Source: CAD feature listing. Evaluate the final solid. Frame: model axes, mm. A direction names the side the tool comes from. Give positions to 0.01 mm unless a question says otherwise; leave off trailing zeros. Write each loop counter-clockwise with the first axis right and the second up, starting at its lowest first coordinate (ties: lowest second). Pieces come first, ordered by that corner, then holes. Notation, with made-up numbers: M -6,-25 L 42,-25 A19 cw 42,3 Z; hole C 74.25,69.25 d10. An arc over 180 degrees is marked long. Return JSON: item names as keys, results as strings.
```python
from build123d import *

# Parameters (mm, degrees)
F1_DEPTH = 3.81
F3_DEPTH = 25.4
F4_R     = 8.724849
F5_DEPTH = 6.35
F7_D     = 15.24


with BuildPart() as f1:
    # F0 (on Top) → F1 (new body)
    with BuildSketch(Plane.XY):
        Polygon((-39.496768, 41.965317), (-39.496768, 35.576135), (-39.496768, -57.938274), (45.595534, -57.938274), (45.595534, 5.372723), (31.655498, 5.372723), (31.655498, 22.507351), (45.595534, 22.507351), (45.595534, 41.965317), align=None)
    extrude(amount=F1_DEPTH)

    # F2 (on face) → F3 (join)
    with BuildSketch(Plane.XY.offset(3.81)):
        Polygon((45.595534, 41.965317), (-39.496768, 41.965317), (-39.496768, -57.938274), (-29.332161, -57.938274), (-29.332161, -15.246916), (45.595534, -15.246916), (45.595534, 5.372723), (31.655498, 5.372723), (31.655498, 22.507351), (45.595534, 22.507351), align=None)
    extrude(amount=F3_DEPTH)

    # F4 (on face) → F5 (join)
    with BuildSketch(Plane.YZ.offset(-29.332161)):
        with Locations((-41.252476, 16.706923)):
            Circle(F4_R)
    extrude(amount=F5_DEPTH)

    # F7 (through all)
    with Locations(Plane.XZ.offset(15.246916)):
        with Locations((21.842908, 16.264843)):
            Hole(F7_D / 2)


solid = f1.part
```
1) Contact query for flat-ended pins moving along their axis: pin 1 Ø6 at (x, z) = (5, 21) entering from -Y; pin 2 Ø8 at (x, y) = (29.5, -37) entering from +Z; pin 3 Ø14 at (y, z) = (-42.5, 17.5) entering from +X. Output: stop coordinate, or through.
Numbers:
{"pin 1": "stops at y = -15.25", "pin 2": "stops at z = 3.81", "pin 3": "stops at x = -22.98"}
2) Cut plane A-A, the plane z = 5.75. Return the cut outline in (x, y).
Numbers:
{"outline": "M -39.5,-57.94 L -29.33,-57.94 L -29.33,-15.25 L 45.6,-15.25 L 45.6,5.37 L 31.66,5.37 L 31.66,22.51 L 45.6,22.51 L 45.6,41.97 L -39.5,41.97 Z"}
3) Set-up query: faces 1 (the face through (-13, -57.938, 3)), 2 (the face through (-22.982, -41, 17)), 3 (the face through (39, 5.373, 14)). Return all of +Z, -Z, +X, -X, +Y, -Y with unobstructed straight access to the full face (end or side cutting, diameter ignored); none if empty.
Numbers:
{"face 1": "+Z, -Z, +X, -X, -Y", "face 2": "+Z, +X, -Y", "face 3": "+Z, -Z, +X"}
4) Cut plane D-D, the plane z = 11. Return the cut outline in (x, y), then the cut area to 3 significant figures.
Numbers:
{"outline": "M -39.5,-57.94 L -29.33,-57.94 L -29.33,-47.85 L -22.98,-47.85 L -22.98,-34.65 L -29.33,-34.65 L -29.33,-15.25 L 16.33,-15.25 L 16.33,41.97 L -39.5,41.97 Z; M 27.35,-15.25 L 45.6,-15.25 L 45.6,5.37 L 31.66,5.37 L 31.66,22.51 L 45.6,22.51 L 45.6,41.97 L 27.35,41.97 Z", "area": "4,520 mm²"}
5) Line query: line 1 (Y direction, x = 37, z = 18.75); line 2 (X direction, y = -39.5, z = 13.75); line 3 (Y direction, x = 11.5, z = 22.25). Output: solid intervals per line, ascending. Write a range as [from, to].
Numbers:
{"line 1": "y = [-15.25, 5.37], [22.51, 41.97]", "line 2": "x = [-39.5, -22.98]", "line 3": "y = [-15.25, 41.97]"}
6) Draft query along Y for faces 4 (the face through (-26.2, -43.14, 8.19)), 5 (the face through (4, 41.965, 14)), 6 (the face through (31.655, 14, 14)), 7 (the face through (45.596, -13, 11)). Return one class per face: released by +Y, released by -Y, zero draft, split by the parting line, or undercut.
Numbers:
{"face 4": "undercut", "face 5": "released by +Y", "face 6": "undercut", "face 7": "zero draft"}
7) Cut plane B-B, the plane x = 36. Return the cut outline in (y, z).
Numbers:
{"outline": "M -57.94,0 L 5.37,0 L 5.37,29.21 L -15.25,29.21 L -15.25,3.81 L -57.94,3.81 Z; M 22.51,0 L 41.97,0 L 41.97,29.21 L 22.51,29.21 Z"}
8) Cut plane C-C, the plane y = -7. Return the cut outline in (x, z), then the cut area to 3 significant figures.
Numbers:
{"outline": "M -39.5,0 L 45.6,0 L 45.6,29.21 L -39.5,29.21 Z; hole C 21.84,16.26 d15.24", "area": "2,300 mm²"}
